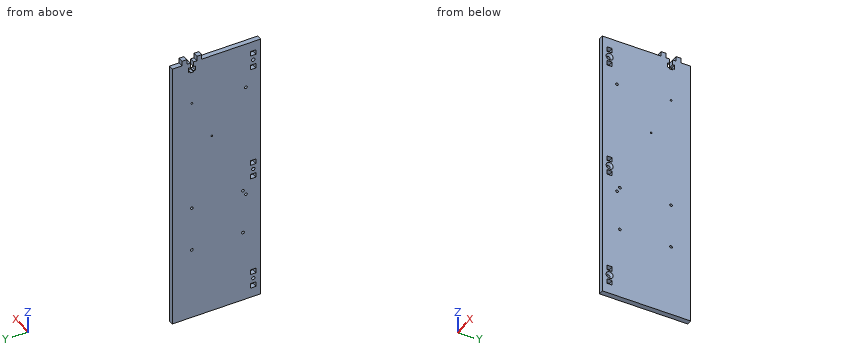
from build123d import *

# Parameters (mm, degrees)
SKETCH1_W                                         = 355.6
SKETCH1_H                                         = 114.3
SKETCH1_R                                         = 2.15265
SKETCH1_W_2                                       = 6.35
SKETCH1_H_2                                       = 6.604
BOSS_EXTRUDE1_DEPTH                               = 6.604
CUT_EXTRUDE1_DEPTH                                = 7.604
SKETCH6_W                                         = 6.35
SKETCH6_H                                         = 6.35
BOSS_EXTRUDE2_DEPTH                               = 6.604
CSK_FOR_8_FLAT_HEAD_SOCKET_CAP_SCREW2_D           = 4.3053
CSK_FOR_8_FLAT_HEAD_SOCKET_CAP_SCREW2_CSINK_D     = 9.1186
CSK_FOR_8_FLAT_HEAD_SOCKET_CAP_SCREW2_CSINK_ANGLE = 82
F_4_40_TAPPED_HOLE2_D                             = 2.2606
F_4_40_TAPPED_HOLE2_DEPTH                         = 7.5946
F_4_40_TAPPED_HOLE2_TIP                           = 0.679152758
F_8_32_TAPPED_HOLE1_D                             = 3.4544
F_8_32_TAPPED_HOLE1_DEPTH                         = 10.7188
F_8_32_TAPPED_HOLE1_TIP                           = 1.037806461
F_8_32_TAPPED_HOLE2_D                             = 3.4544
F_8_32_TAPPED_HOLE2_DEPTH                         = 10.7188
F_8_32_TAPPED_HOLE2_TIP                           = 1.037806461


with BuildPart() as part:
    # Sketch1 → Boss-Extrude1 (new body)
    with BuildSketch(Plane(origin=(0, 0, 0), x_dir=(0, 0, -1), z_dir=(1, 0, 0))):
        with Locations((0, 57.15)):
            Rectangle(SKETCH1_W, SKETCH1_H)
        with Locations((-152.4, 9.525)):
            Circle(SKETCH1_R, mode=Mode.SUBTRACT)
        with Locations((0, 9.525)):
            Circle(SKETCH1_R, mode=Mode.SUBTRACT)
        with Locations((152.4, 9.525)):
            Circle(SKETCH1_R, mode=Mode.SUBTRACT)
        with Locations((-142.875, 9.525)):
            Rectangle(SKETCH1_W_2, SKETCH1_H_2, mode=Mode.SUBTRACT)
        with Locations((-161.925, 9.525)):
            Rectangle(SKETCH1_W_2, SKETCH1_H_2, mode=Mode.SUBTRACT)
        with Locations((9.525, 9.525)):
            Rectangle(SKETCH1_W_2, SKETCH1_H_2, mode=Mode.SUBTRACT)
        with Locations((-9.525, 9.525)):
            Rectangle(SKETCH1_W_2, SKETCH1_H_2, mode=Mode.SUBTRACT)
        with Locations((161.925, 9.525)):
            Rectangle(SKETCH1_W_2, SKETCH1_H_2, mode=Mode.SUBTRACT)
        with Locations((142.875, 9.525)):
            Rectangle(SKETCH1_W_2, SKETCH1_H_2, mode=Mode.SUBTRACT)
    extrude(amount=BOSS_EXTRUDE1_DEPTH)

    # Sketch5 → Cut-Extrude1 (cut, through all)
    with BuildSketch(Plane.ZY):
        Polygon((177.8, 90.9828), (171.45, 90.9828), (171.45, 93.2688), (165.5064, 93.2688), (165.5064, 90.9828), (163.83, 90.9828), (163.83, 86.8172), (165.5064, 86.8172), (165.5064, 84.5312), (171.45, 84.5312), (171.45, 86.8172), (177.8, 86.8172), align=None)
    extrude(amount=-CUT_EXTRUDE1_DEPTH, mode=Mode.SUBTRACT)

    # Sketch6 → Boss-Extrude2 (add)
    with BuildSketch(Plane.ZY):
        with Locations((180.975, 98.425)):
            Rectangle(SKETCH6_W, SKETCH6_H)
        with Locations((180.975, 79.375)):
            Rectangle(SKETCH6_W, SKETCH6_H)
    extrude(amount=-BOSS_EXTRUDE2_DEPTH)

    # CSK for #8 Flat Head Socket Cap Screw2 (through all)
    with Locations(Plane(origin=(6.604, 0, 0), x_dir=(0, 0, -1), z_dir=(1, 0, 0))):
        with Locations((-152.4, 9.525), (0, 9.525), (152.4, 9.525)):
            CounterSinkHole(CSK_FOR_8_FLAT_HEAD_SOCKET_CAP_SCREW2_D / 2, CSK_FOR_8_FLAT_HEAD_SOCKET_CAP_SCREW2_CSINK_D / 2, counter_sink_angle=CSK_FOR_8_FLAT_HEAD_SOCKET_CAP_SCREW2_CSINK_ANGLE)

    # #4-40 Tapped Hole2
    with Locations(Plane.ZY):
        with Locations((120.65, 88.9), (66.04, 63.2968)):
            Hole(F_4_40_TAPPED_HOLE2_D / 2, depth=F_4_40_TAPPED_HOLE2_DEPTH)
            with Locations((0, 0, -(F_4_40_TAPPED_HOLE2_DEPTH + F_4_40_TAPPED_HOLE2_TIP / 2))):  # 118° drill point
                Cone(0, F_4_40_TAPPED_HOLE2_D / 2, F_4_40_TAPPED_HOLE2_TIP, mode=Mode.SUBTRACT)

    # #8-32 Tapped Hole1
    with Locations(Plane.ZY):
        with Locations((-83.82, 88.9), (-25.4, 88.9), (-83.82, 22.86), (-25.4, 22.86)):
            Hole(F_8_32_TAPPED_HOLE1_D / 2, depth=F_8_32_TAPPED_HOLE1_DEPTH)
            with Locations((0, 0, -(F_8_32_TAPPED_HOLE1_DEPTH + F_8_32_TAPPED_HOLE1_TIP / 2))):  # 118° drill point
                Cone(0, F_8_32_TAPPED_HOLE1_D / 2, F_8_32_TAPPED_HOLE1_TIP, mode=Mode.SUBTRACT)

    # #8-32 Tapped Hole2
    with Locations(Plane(origin=(6.604, 0, 0), x_dir=(0, 0, -1), z_dir=(1, 0, 0))):
        with Locations((-117.475, 19.05), (31.75, 19.05)):
            Hole(F_8_32_TAPPED_HOLE2_D / 2, depth=F_8_32_TAPPED_HOLE2_DEPTH)
            with Locations((0, 0, -(F_8_32_TAPPED_HOLE2_DEPTH + F_8_32_TAPPED_HOLE2_TIP / 2))):  # 118° drill point
                Cone(0, F_8_32_TAPPED_HOLE2_D / 2, F_8_32_TAPPED_HOLE2_TIP, mode=Mode.SUBTRACT)


solid = part.part
Build history of the part. All positions in model axes, mm. Round coordinates to 2 decimals unless told otherwise and drop trailing zeros. Write each loop counter-clockwise with the first axis right and the second up, starting at its lowest first coordinate (ties: lowest second). Pieces come first, ordered by that corner, then holes. Notation, with made-up numbers: M 30,26 L 48,26 A33 ccw 48,64 Z; hole C 12,69 d4. An arc over 180 degrees is marked long. Answer in a Markdown table with one row per item.
1. Flat gauge pins, fed straight in: P1, Ø2, axis at x = 4.5, y = 8.5, coming from the +Z side; P2, Ø2, axis at y = 88.9, z = -25.4, coming from the -X side. Where does each tip first touch, or does it go through?
Geometry check:
| item | result |
|---|---|
| P1 | z = 177.8 |
| P2 | through |
2. Probe L1, parallel to Z at x = 2, y = 88.9; L2, parallel to Y at x = 2, z = -83.82; L3, parallel to Z at x = 6, y = 22.5. List the from-to ranges inside material, lowest first. Write a range as [from, to].
Geometry check:
| item | result |
|---|---|
| L1 | [-177.8, -85.55], [-82.09, -27.13], [-23.67, 119.52], [121.78, 163.83] |
| L2 | [0, 21.13], [24.59, 87.17], [90.63, 114.3] |
| L3 | [-177.8, -85.51], [-82.13, -27.09], [-23.71, 177.8] |
3. Saw through at A-A (y = 41). List the corners of the cut face in (x, z), and give its area (3 significant figures).
Geometry check:
| item | result |
|---|---|
| outline | M 0,-177.8 L 6.6,-177.8 L 6.6,177.8 L 0,177.8 Z |
| area | 2,350 mm2 |
4. Saw through at B-B (x = 2.75). State how many separate pieces and enclosed holes the cut face has, and give its area (3 significant figures).
Geometry check:
| item | result |
|---|---|
| separate pieces | 1 |
| enclosed holes | 17 |
| area | 40,300 mm2 |
